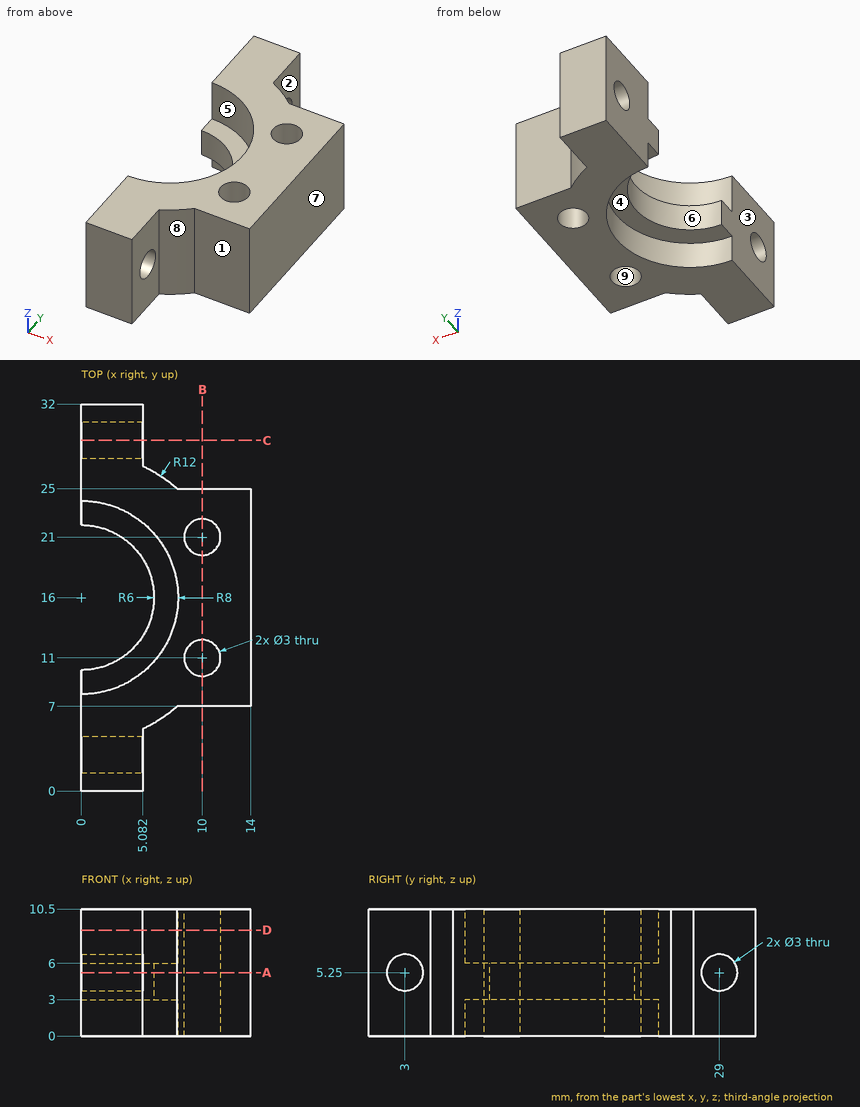
Verification items for this drawing (mm, ordinates from the low corner). A direction names the side the tool comes from. Give positions to 0.01 mm unless a question says otherwise; leave off trailing zeros. Loops run counter-clockwise (first coordinate to the right, second up) from the corner with the lowest first, then second, coordinate; pieces in that order, holes last. Notation, with made-up numbers: M -26,0 L 6,0 A10 cw 6,5 Z; hole C -20.75,-31 d4. An arc over 180 degrees is marked long. Write each question's results on one line, items separated by ' | '.
1) Section check C-C, the plane y = 29. Record the boundary of the cut face in (x, z).
Answers follow:
outline: M 0,0 L 5.08,0 L 5.08,3.75 L 0,3.75 Z; M 0,6.75 L 5.08,6.75 L 5.08,10.5 L 0,10.5 Z
2) Tool access check on the marked faces 1, 2, 3, 4 and 5. Record the directions out of +Z, -Z, +X, -X, +Y, -Y that give a thin tool (end or side, any length) a straight path to the whole face; none if there is none.
Answers follow:
face 1: +Z, -Z, +X, -Y | face 2: +Z, -Z, +X, +Y | face 3: +Z, -Z, -X, +Y, -Y | face 4: -Z, -X | face 5: +Z, -X
3) Section check A-A, the plane z = 5.25. Record the boundary of the cut face in (x, y).
Answers follow:
outline: M 0,0 L 5.08,0 L 5.08,1.5 L 0,1.5 Z; M 0,4.5 L 5.08,4.5 L 5.08,5.13 A12 ccw 7.94,7 L 14,7 L 14,25 L 7.94,25 A12 ccw 5.08,26.87 L 5.08,27.5 L 0,27.5 L 0,22 A6 cw 0,10 Z; M 0,30.5 L 5.08,30.5 L 5.08,32 L 0,32 Z; hole C 10,11 d3; hole C 10,21 d3
4) Section check D-D, the plane z = 8.75. Record the boundary of the cut face in (x, y).
Answers follow:
outline: M 0,0 L 5.08,0 L 5.08,5.13 A12 ccw 7.94,7 L 14,7 L 14,25 L 7.94,25 A12 ccw 5.08,26.87 L 5.08,32 L 0,32 L 0,24 A8 cw 0,8 Z; hole C 10,11 d3; hole C 10,21 d3
5) Release check for a two-part mould opening along Y. For the marked faces 6, 7, 8 and 9 record: +Y half, -Y half, draft (parallel to the pull), parting line (faces both ways), or undercut.
Answers follow:
face 6: undercut | face 7: draft | face 8: -Y half | face 9: undercut
6) Section check B-B, the plane x = 10. Record the boundary of the cut face in (y, z).
Answers follow:
outline: M 7,0 L 9.5,0 L 9.5,10.5 L 7,10.5 Z; M 12.5,0 L 19.5,0 L 19.5,10.5 L 12.5,10.5 Z; M 22.5,0 L 25,0 L 25,10.5 L 22.5,10.5 Z
7) Gauge pin test, flat ends, axial feed: pin 1 (3.5 mm diameter, centred on x = 10, y = 11, fed in from +Z); pin 2 (1.5 mm diameter, centred on y = 1.5, z = 5.5, fed in from +X); pin 3 (5 mm diameter, centred on x = 12, z = 4.5, fed in from +Y); pin 4 (5 mm diameter, centred on x = 11, z = 8, fed in from -Y). Record the tip position at first contact, or that the pin passes through.
Answers follow:
pin 1: z = 10.5 | pin 2: x = 5.08 | pin 3: y = 25 | pin 4: y = 7
8) Thickness scan on line 1 (Y direction, x = 10, z = 3); line 2 (Y direction, x = 3, z = 4) (1 decimal); line 3 (Y direction, x = 11, z = 9). Record the ranges inside material, lowest first.
Answers follow:
line 1: 7 to 9.5, 12.5 to 19.5, 22.5 to 25 | line 2: 0 to 2.2, 3.8 to 10.8, 21.2 to 28.2, 29.8 to 32 | line 3: 7 to 9.88, 12.12 to 19.88, 22.12 to 25
